Design review of the part built by this model. Coordinates are the model's own, in mm. A direction names the side the tool comes from. Coordinates: 2 decimals unless noted, no trailing zeros. Order: outer loops, then holes, each group sorted by start corner. A loop starts at its lowest first (then second) coordinate and runs counter-clockwise, first axis right, second up. Notation, with made-up numbers: (-26.75, 48.5) -> (-14.75, 48.5) arc R23 cw to (-14.75, 63.5) -> close; hole circle Ø11 at (-33.5, 12.25). An arc over 180 degrees is marked (long way). Use a Markdown table: item, result. Add a question column.
Q1. Add section C-C (x = -32). State the section outline as (y, z) points (3 decimals).
Q2. Machinability: for faces 1 (the face through (-44.347, 112.217, 1.61)), 2 (the face through (-48.502, 124.072, 1.565)), which of the approach directions +Z, -Z, +X, -X, +Y, -Y give a long, thin tool a straight path to every point of the face, cutting with its end or side? Answer none if there is none.
Q3. Add section D-D (x = 41). State the section outline as (y, z) points (3 decimals), then the cut area to 3 significant figures.
Q4. Wall thickness on probe 1 along X at (y, z) = (115.5, 0.75); probe 2 along X at (y, z) = (116, 2.05); probe 3 along Y at (x, z) = (11, 0.6): over which ranges is each line inside the solid? List them lowest first.
Q5. Add section B-B (z = 1.9). Count the separate pieces of the cut face and the enclosed holes in it, then the cut area to 3 significant figures.
Q6. The part is to be moulded in two halves that separate along Y. For faces 3 (the face through (0, 137.186, 2)), 4 (the face through (52.425, 117, 2)), 5 (the face through (-34.67, 122.46, 1.61)), say which applies: pulls with the +Y half, pulls with the -Y half, needs draft (parallel to the pull), parting line crosses it, or undercut.
Q7. Insertion check: pin 1 (1 mm diameter, centred on x = -27, z = 0.5, fed in from +Y); pin 2 (1 mm diameter, centred on x = -1, z = 2.5, fed in from -Y). Each pin has a flat end and moves straight along its axis. Give the tip position at first contact, or say it passes through.
Q8. Add section A-A (x = 1). State the section outline as (y, z) points (3 decimals).
Autodesk Inventor part; units mm, degrees
ref_plane "YZ Plane" through (0, 0, 0) normal (1, 0, 0) x (0, 1, 0)
ref_plane "XZ Plane" through (0, 0, 0) normal (0, 1, 0) x (-1, 0, 0)
ref_plane "XY Plane" through (0, 0, 0) normal (0, 0, 1) x (1, 0, 0)
sketch "Base" plane through (0, 0, 0) normal (0, 0, 1) x (1, 0, 0)
  circle A0 centre (-46.4246, 117.9827) radius 2.5
  line L0 (-52.4246, 120.7805) -> (-52.4246, 111.9827)
  line L1 (-52.4246, 111.9827) -> (-44.2408, 111.9827)
  line L2 (-52.4246, 120.7805) -> (-45.3975, 126.677)
  line L3 (-45.3975, 126.677) -> (-16.5235, 137.1863)
  line L4 (-44.2408, 111.9827) -> (-39.3049, 116.1244)
  line L5 (-39.3049, 116.1244) -> (-11.6601, 126.1863)
  line L6 (-11.6601, 126.1863) -> (0.0157, 126.1863)
  line L7 (-16.5235, 137.1863) -> (0, 137.1863)
  line L8 (0.0001, 252.4162) -> (0.0001, -227.6975)
  line L9 (52.4249, 120.7805) -> (52.4249, 111.9827)
  line L10 (52.4249, 111.9827) -> (44.2411, 111.9827)
  line L11 (52.4249, 120.7805) -> (45.3977, 126.677)
  line L12 (44.2411, 111.9827) -> (39.3052, 116.1244)
  line L13 (39.3052, 116.1244) -> (11.6604, 126.1863)
  line L14 (11.6604, 126.1863) -> (0.0157, 126.1863)
  line L15 (16.5238, 137.1863) -> (0, 137.1863)
  line L16 (16.5238, 137.1863) -> (45.3977, 126.677)
  ellipse E0 centre (-12.7181, 132.1863) end of major axis (-10.7181, 132.1863) minor radius 1.9897 construction
  ellipse E1 centre (12.7183, 132.1863) end of major axis (14.7183, 132.1863) minor radius 1.9897 construction
  circle A1 centre (-46.4246, 117.9827) radius 3.175
  circle A2 centre (46.4246, 117.9827) radius 3.175
  point P0 (0, 0)
  dimension "d1" = 5
  dimension "d2" = 6
  dimension "d3" = 6
  dimension "d5" = 12
  dimension "d6" = 160
  dimension "d7" = 160
  dimension "d8" = 6
  dimension "d9" = 6
  dimension "d10" = 6
  dimension "d11" = 6
  dimension "d20" = 5
extrude "Plate1" add sketch "Base" along normal blind 3.175 contours L2 L3 L7 L8 L6 L5 L4 L1 L0 | L15 L16 L11 L9 L10 L12 L13 L14 L6 L8
fillet "FilletsFeature" radius 4 14 edges at (-45.3975, 126.677, 1.5875) (-16.5235, 137.1863, 1.5875) (-52.4246, 120.7805, 1.5875) (-52.4246, 111.9827, 1.5875) (16.5238, 137.1863, 1.5875) (45.3977, 126.677, 1.5875) (52.4249, 120.7805, 1.5875) (52.4249, 111.9827, 1.5875) (44.2411, 111.9827, 1.5875) (39.3052, 116.1244, 1.5875) (11.6604, 126.1863, 1.5875) (-11.6601, 126.1863, 1.5875) (-39.3049, 116.1244, 1.5875) (-44.2408, 111.9827, 1.5875)
ref_plane "BentCutPlane" through (-12.7181, 132.4436, 8.3161) normal (0, 0.1014, 0.9948) x (0, -0.9948, 0.1014)
sketch "BentCutProfile" plane through (-12.7181, 132.4436, 8.3161) normal (0, 0.1014, 0.9948) x (0, -0.9948, 0.1014)
  circle A0 centre (0, 0) radius 2
  circle A1 centre (0, 25.4364) radius 2
  point P0 (130.9175, 12.7181)
hole "BentCutProfileHoleFeature" at (-12.7181, 132.4436, 8.3161) at (12.7183, 132.4436, 8.3161) direction (0, -0.1014, -0.9948) diameter 4.5 end through all
sketch "UtilityHoles" plane through (0, 0, 0) normal (0, 0, -1) x (-1, 0, 0)
  ellipse E0 centre (-12.7183, 131.5959) end of major axis (-12.7183, 129.3342) minor radius 2.25
  ellipse E1 centre (12.7181, 131.5959) end of major axis (12.7181, 129.3342) minor radius 2.25
  circle A0 centre (-46.4246, 117.9827) radius 3.175
  line L0 (15.8182, 137.1863) -> (-15.8185, 137.1863)
  line L1 (-0.0001, 137.1863) -> (-0.0001, 126.1863)
  line L2 (10.9548, 126.1863) -> (-10.9551, 126.1863)
  line L3 (-12.7183, 131.5959) -> (-44.1201, 120.1666) construction
  line L4 (-12.3232, 125.945) -> (-38.6424, 116.3656)
  line L5 (-12.7183, 131.5959) -> (12.7181, 131.5959) construction
  circle A1 centre (-0.0001, 131.5959) radius 2
  circle A2 centre (-24.6696, 127.246) radius 2
  circle A3 centre (-36.6208, 122.8961) radius 2
  circle A4 centre (24.6693, 127.246) radius 2
  circle A5 centre (36.6205, 122.8961) radius 2
  point P0 (0, 0)
  dimension "d21" = 4
  dimension "d22" = 12.7182
  dimension "d23" = 12.7182
  dimension "d24" = 12.7182
hole "UtilityHolesFeature" at (36.6208, 122.8961, 0) at (24.6696, 127.246, 0) at (0.0001, 131.5959, 0) at (-24.6693, 127.246, 0) at (-36.6205, 122.8961, 0) direction (0, 0, 1) diameter 4 end through all
equation "\"d18\" = Thickness"
equation "\"d23\" = d22"
equation "\"d24\" = d22"
equation "\"d30\" = Thickness"
equation "\"d0\" = Thickness"
equation "\"BendRadius\" = Thickness"
equation "\"BendReliefWidth\" = Thickness"
equation "\"BendReliefDepth\" = 0.5 * Thickness"
equation "\"CornerReliefSize\" = 4 * Thickness"
equation "\"MinimumRemnant\" = 2 * Thickness"
equation "\"TransitionRadius\" = BendRadius"
equation "\"JacobiRadiusSize\" = BendRadius"
equation "\"GapSize\" = Thickness"
properties part number "HeadTopConnector"
Established:
| question | item | result |
|---|---|---|
| 1 | outline | (118.783, 0) -> (131.553, 0) -> (131.553, 3.175) -> (118.783, 3.175) -> close |
| 2 | face 1 | +Z, -Z, -Y |
| 2 | face 2 | +Z, -Z, -X, +Y |
| 3 | outline | (114.702, 0) -> (128.278, 0) -> (128.278, 3.175) -> (114.702, 3.175) -> close |
| 3 | area | 43.1 mm^2 |
| 4 | probe 1 | -52.4 to -48.4, -44.45 to -40.05, 40.05 to 44.45, 48.4 to 52.4 |
| 4 | probe 2 | -52.42 to -48.9, -43.94 to -39.39, 39.39 to 43.94, 48.9 to 52.42 |
| 4 | probe 3 | 126.19 to 130.2, 133.12 to 137.19 |
| 5 | separate pieces | 1 |
| 5 | enclosed holes | 9 |
| 5 | area | 1,120 mm^2 |
| 6 | face 3 | pulls with the +Y half |
| 6 | face 4 | needs draft |
| 6 | face 5 | undercut |
| 7 | pin 1 | y = 133.56 |
| 7 | pin 2 | y = 126.19 |
| 8 | outline | (126.186, 0) -> (129.864, 0) -> (129.864, 3.175) -> (126.186, 3.175) -> close; (133.328, 0) -> (137.186, 0) -> (137.186, 3.175) -> (133.328, 3.175) -> close |
